Part model, mm, in its own coordinate system. Face numbers are marked on the shaded views. Round coordinates to 2 decimals unless told otherwise and drop trailing zeros. Order: outer loops, then holes, each group sorted by start corner. A loop starts at its lowest first (then second) coordinate and runs counter-clockwise, first axis right, second up. Notation, with made-up numbers: (72, 20.5) - (113, 20.5) arc R33 cw to (113, 57.5) - close; hole circle Ø2 at (52, -0.75). An arc over 180 degrees is marked (long way). Return JSON: item names as keys, results as strings. Group by question number.
Item 1: Drop a flat-ended pin along its axis: pin 1 (0.6 mm diameter, centred on y = -3, z = 0, fed in from +X) (3 decimals). Give the stop position or say it passes through.
Item 2: Two-plate mould, pull along Y, no slides. Class the marked faces 1 and 2: released by +Y, released by -Y, zero draft, split by the parting line, or undercut.
Item 3: Saw through at B-B on x = 2.75. List the corners of the cut face in (y, z).
Item 4: Saw through at A-A on y = -8.2. List the corners of the cut face in (x, z) (3 decimals), and give its area (3 significant figures).
Item 5: Probe probe 1 along Z at (x, y) = (1, 2.5); probe 2 along Z at (x, y) = (5.5, 12.5); probe 3 along Y at (x, z) = (2, 2.95). List the from-to ranges inside material, lowest first.
Item 6: Saw through at C-C on z = 3.6. List the corners of the cut face in (x, y).
Item 7: Saw through at D-D on x = 0. List the corners of the cut face in (y, z).
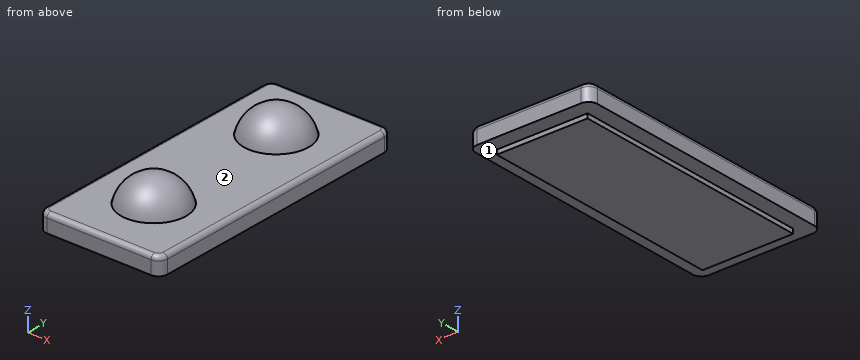
```python
from build123d import *

# Parameters (mm, degrees)
SKETCH1_W           = 10.25
SKETCH1_H           = 27.5
BOSS_EXTRUDE1_DEPTH = 0.5
SKETCH2_W           = 13.75
SKETCH2_H           = 31
BOSS_EXTRUDE2_DEPTH = 2
FILLET1_R           = 1
FILLET2_R           = 0.5
SKETCH3_R           = 3.65
CUT_EXTRUDE1_DEPTH  = 0.1


# Read off the part's stored shape, not the designer's step: Dome1, Dome2
with BuildPart() as part:
    # Sketch1 → Boss-Extrude1 (new body)
    with BuildSketch(Plane.XY):
        Rectangle(SKETCH1_W, SKETCH1_H)
    extrude(amount=BOSS_EXTRUDE1_DEPTH)

    # Sketch2 → Boss-Extrude2 (add)
    with BuildSketch(Plane.XY.offset(0.5)):
        Rectangle(SKETCH2_W, SKETCH2_H)
    extrude(amount=BOSS_EXTRUDE2_DEPTH)

    # Fillet1
    fillet1_edges = [part.edges().sort_by_distance(p)[0] for p in [
        (6.875, -15.5, 1.5),
        (6.875, 15.5, 1.5),
        (-6.875, 15.5, 1.5),
        (-6.875, -15.5, 1.5),
    ]]
    fillet(fillet1_edges, radius=FILLET1_R)

    # Fillet2
    fillet2_edges = [part.edges().sort_by_distance(p)[0] for p in [
        (0, 15.5, 2.5),
        (6.875, 0, 2.5),
        (-6.875, 0, 2.5),
        (0, -15.5, 2.5),
        (-6.582106781, 15.207106781, 2.5),
        (-6.582106781, -15.207106781, 2.5),
        (6.582106781, -15.207106781, 2.5),
        (6.582106781, 15.207106781, 2.5),
    ]]
    fillet(fillet2_edges, radius=FILLET2_R)

    # Sketch3 → Cut-Extrude1 (cut)
    with BuildSketch(Plane.XY.offset(2.5)):
        with Locations((0, 8.2)):
            Circle(SKETCH3_R)
    cut_extrude1 = extrude(amount=-CUT_EXTRUDE1_DEPTH, mode=Mode.SUBTRACT)

    # Mirror1: Cut-Extrude1 across plane
    add(cut_extrude1.mirror(Plane.ZX), mode=Mode.SUBTRACT)

    # Dome1 outline → Dome1 (revolve)
    with BuildSketch(Plane.XZ.offset(-8.2)):
        with BuildLine():
            Line((0, 2.4), (3.650000001, 2.399999996))
            ThreePointArc((3.650000001, 2.399999996), (2.362334652, 4.553757157), (0, 5.4))
            Line((0, 5.4), (0, 2.4))
        make_face()
    revolve(axis=Axis((0, 8.2, 0), (0, 0, 1)))

    # Dome2 outline → Dome2 (revolve)
    with BuildSketch(Plane.XZ.offset(8.2)):
        with BuildLine():
            Line((0, 2.4), (3.650000001, 2.399999996))
            ThreePointArc((3.650000001, 2.399999996), (2.362334652, 4.553757157), (0, 5.4))
            Line((0, 5.4), (0, 2.4))
        make_face()
    revolve(axis=Axis((0, -8.2, 0), (0, 0, 1)))


solid = part.part
```
Filled in:
{
 "1": {"pin 1": "stops at x = 5.125"},
 "2": {"face 1": "zero draft", "face 2": "undercut"},
 "3": {"outline": "(-15.5, 0.5) - (-13.75, 0.5) - (-13.75, 0) - (13.75, 0) - (13.75, 0.5) - (15.5, 0.5) - (15.5, 2) arc R0.5 ccw to (15, 2.5) - (10.6, 2.5) - (10.6, 2.4) arc R2.51 ccw to (5.8, 2.4) - (5.8, 2.5) - (-5.8, 2.5) - (-5.8, 2.4) arc R2.51 ccw to (-10.6, 2.4) - (-10.6, 2.5) - (-15, 2.5) arc R0.5 ccw to (-15.5, 2) - close"},
 "4": {"outline": "(-6.875, 0.5) - (-5.125, 0.5) - (-5.125, 0) - (5.125, 0) - (5.125, 0.5) - (6.875, 0.5) - (6.875, 2) arc R0.5 ccw to (6.375, 2.5) - (3.65, 2.5) - (3.65, 2.4) arc R3.72 ccw to (-3.65, 2.4) - (-3.65, 2.5) - (-6.375, 2.5) arc R0.5 ccw to (-6.875, 2) - close", "area": "48.2 mm^2"},
 "5": {"probe 1": "z = 0 to 2.5", "probe 2": "z = 0.5 to 2.5", "probe 3": "y = -11.07 to -5.33, 5.33 to 11.07"},
 "6": {"outline": "circle Ø6.37 at (0, -8.2); circle Ø6.37 at (0, 8.2)"},
 "7": {"outline": "(-15.5, 0.5) - (-13.75, 0.5) - (-13.75, 0) - (13.75, 0) - (13.75, 0.5) - (15.5, 0.5) - (15.5, 2) arc R0.5 ccw to (15, 2.5) - (11.85, 2.5) - (11.85, 2.4) arc R3.72 ccw to (4.55, 2.4) - (4.55, 2.5) - (-4.55, 2.5) - (-4.55, 2.4) arc R3.72 ccw to (-11.85, 2.4) - (-11.85, 2.5) - (-15, 2.5) arc R0.5 ccw to (-15.5, 2) - close"}
}
